```python
from build123d import *

# Parameters (mm, degrees)
F0_W     = 13
F0_H     = 10
F1_DEPTH = 15
F2_W     = 8
F2_H     = 6
F3_DEPTH = 25
F4_W     = 6
F4_H     = 7
F5_DEPTH = 13
F6_R     = 1


with BuildPart() as f1:
    # F0 (on Top) → F1 (new body)
    with BuildSketch(Plane.XY):
        Rectangle(F0_W, F0_H)
    extrude(amount=F1_DEPTH)

    # F2 (on face) → F3 (cut)
    with BuildSketch(Plane.XY.offset(15)):
        Rectangle(F2_W, F2_H)
    extrude(amount=-F3_DEPTH, mode=Mode.SUBTRACT)

    # F4 (on face) → F5 (cut)
    with BuildSketch(Plane(origin=(-6.5, 0, 0), x_dir=(0, -1, 0), z_dir=(-1, 0, 0))):
        with Locations((0, 9)):
            Rectangle(F4_W, F4_H)
    extrude(amount=-F5_DEPTH, mode=Mode.SUBTRACT)

    # F6
    f6_edges = [f1.edges().sort_by_distance(p)[0] for p in [
        (4, 0, 0),
        (0, 3, 0),
        (-4, 0, 0),
        (0, -3, 0),
    ]]
    fillet(f6_edges, radius=F6_R)


solid = f1.part
```
Build history of the part. All positions in model axes, mm. A direction names the side the tool comes from. Give positions to 0.01 mm unless a question says otherwise; leave off trailing zeros. Loops run counter-clockwise (first coordinate to the right, second up) from the corner with the lowest first, then second, coordinate; pieces in that order, holes last.
Item 1: Slice it at A-A, the plane z = 9.5. List the corners of the cut face in (x, y), and give its area (3 significant figures).
Answers follow:
outline: (-6.5, -5) - (6.5, -5) - (6.5, -3) - (-6.5, -3) - close; (-6.5, 3) - (6.5, 3) - (6.5, 5) - (-6.5, 5) - close
area: 52.0 mm2
Item 2: Pull direction Z, two halves, no side cores. Call faces 1 (the face through (-4.301, 0.056, 0.285)), 2 (the face through (-5, 0, 5.5)), 3 (the face through (0, 5, 7)): released by +Z, released by -Z, zero draft, split by the parting line, or undercut.
Answers follow:
face 1: released by -Z
face 2: undercut
face 3: zero draft
Item 3: Slice it at C-C, the plane x = 1. List the corners of the cut face in (y, z), and give its area (3 significant figures).
Answers follow:
outline: (-5, 0) - (-4, 0) arc R1 ccw to (-3, 1) - (-3, 15) - (-5, 15) - close; (3, 1) arc R1 ccw to (4, 0) - (5, 0) - (5, 15) - (3, 15) - close
area: 59.6 mm2
Item 4: Which spindle directions (+Z, -Z, +X, -X, +Y, -Y) get a long thin tool onto all of the face, cutting with end or side? Do faces 4 (the face through (4, 0, 3)), 5 (the face through (-6.5, 0, 4)), 6 (the face through (0, 3, 8)), 7 (the face through (5, 0, 5.5)), 8 (the face through (0.07, 3.301, 0.285)). Say none if no direction does.
Answers follow:
face 4: +Z, -Z
face 5: +Z, -Z, -X, +Y, -Y
face 6: none
face 7: +X, -X
face 8: -Z
Item 5: Slice it at D-D, the plane z = 2.25. List the corners of the cut face in (x, y), and give its area (3 significant figures).
Answers follow:
outline: (-6.5, -5) - (6.5, -5) - (6.5, 5) - (-6.5, 5) - close; hole (-4, -3) - (4, -3) - (4, 3) - (-4, 3) - close
area: 82.0 mm2
Item 6: Slice it at B-B, the plane y = 1.25. List the corners of the cut face in (x, z), and give its area (3 significant figures).
Answers follow:
outline: (-6.5, 0) - (-5, 0) arc R1 ccw to (-4, 1) - (-4, 5.5) - (-6.5, 5.5) - close; (-6.5, 12.5) - (-4, 12.5) - (-4, 15) - (-6.5, 15) - close; (4, 1) arc R1 ccw to (5, 0) - (6.5, 0) - (6.5, 5.5) - (4, 5.5) - close; (4, 12.5) - (6.5, 12.5) - (6.5, 15) - (4, 15) - close
area: 39.6 mm2
Item 7: Drill centre lines: line 1 (Y direction, x = 0, z = 7.75); line 2 (X direction, y = -1, z = 5.25); line 3 (Z direction, x = -4.75, y = 0.75). Where is each one in solid material? Low to high.
Answers follow:
line 1: y = -5 to -3, 3 to 5
line 2: x = -6.5 to -4, 4 to 6.5
line 3: z = 0.03 to 5.5, 12.5 to 15
